Print and shaded views of the part. All mm, measured from the part's lowest x, y and z. A direction names the side the tool comes from. Coordinates: 2 decimals unless noted, no trailing zeros. Order: outer loops, then holes, each group sorted by start corner. A loop starts at its lowest first (then second) coordinate and runs counter-clockwise, first axis right, second up. Notation, with made-up numbers: M 27,44.25 L 31,44.25 A7 ccw 31,50.25 Z; hole C -27,50 d3. An arc over 180 degrees is marked long. Return JSON: item names as keys, results as strings.
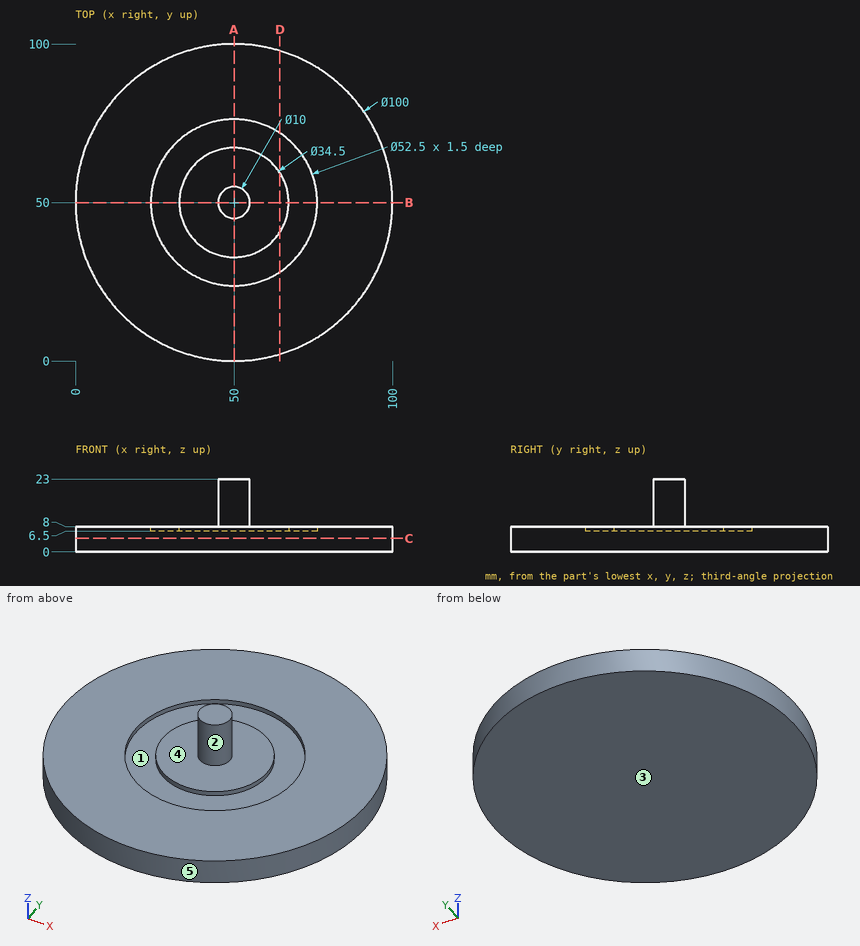
Item 1: Drop flat-ended pins along their axis: pin 1 Ø12 at (x, z) = (55, 9.5) entering from -Y; pin 2 Ø8 at (y, z) = (21, 14.5) entering from -X; pin 3 Ø4 at (x, z) = (31.5, 5.5) entering from +Y; pin 4 Ø1.5 at (y, z) = (68, 2.5) entering from +X. Give the stop position or say it passes through.
Check result:
{"pin 1": "stops at y = 0", "pin 2": "passes through", "pin 3": "stops at y = 97.2", "pin 4": "stops at x = 96.93"}
Item 2: Wall check: line 1 (Y direction, x = 50, z = 7.1); line 2 (Z direction, x = 66.5, y = 12); line 3 (Y direction, x = 34, z = 2.75). Give the ranges that are in metal, low to high.
Check result:
{"line 1": "y = 0 to 23.75, 32.75 to 67.25, 76.25 to 100", "line 2": "z = 0 to 8", "line 3": "y = 2.63 to 97.37"}
Item 3: Saw through at C-C (z = 4.25). Write the cut outline in (x, y), and give its area (3 significant figures).
Check result:
{"outline": "C 50,50 d100", "area": "7,850 mm2"}
Item 4: 3-axis set-ups, long thin cutter, end or side, ignore diameter. For the marked faces 4 and 5: which of +Z, -Z, +X, -X, +Y, -Y reach the whole face in a straight line?
Check result:
{"face 4": "+Z", "face 5": "+Z, -Z"}
Item 5: Pull direction X, two halves, no side cores. Call the marked faces 1, 2 and 3: +X half, -X half, draft (parallel to the pull), parting line (faces both ways), or undercut.
Check result:
{"face 1": "undercut", "face 2": "parting line", "face 3": "draft"}
Item 6: Saw through at D-D (x = 64.5). Write the cut outline in (y, z).
Check result:
{"outline": "M 2.15,0 L 97.85,0 L 97.85,8 L 71.88,8 L 71.88,6.5 L 59.34,6.5 L 59.34,8 L 40.66,8 L 40.66,6.5 L 28.12,6.5 L 28.12,8 L 2.15,8 Z"}
Item 7: Saw through at A-A (x = 50). Write the cut outline in (y, z), and give its area (3 significant figures).
Check result:
{"outline": "M 0,0 L 100,0 L 100,8 L 76.25,8 L 76.25,6.5 L 67.25,6.5 L 67.25,8 L 55,8 L 55,23 L 45,23 L 45,8 L 32.75,8 L 32.75,6.5 L 23.75,6.5 L 23.75,8 L 0,8 Z", "area": "923 mm2"}
